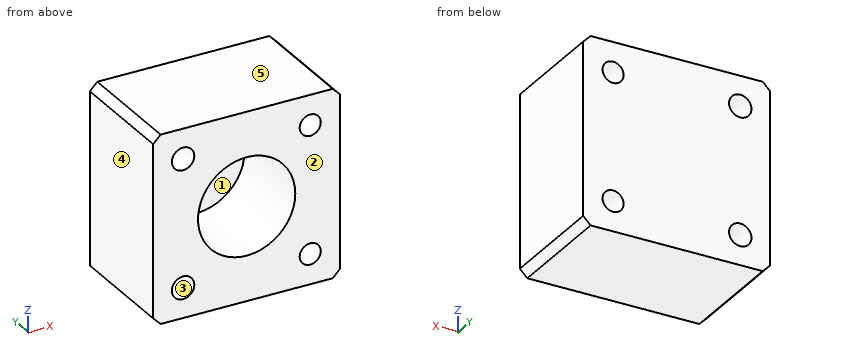
```python
from build123d import *

# Parameters (mm, degrees)
F0_W     = 125
F0_H     = 125
F1_DEPTH = 75
F2_SIZE  = 5
F3_R     = 7.5
F3_R_2   = 7.043913
F4_DEPTH = 75.001
F5_R     = 32.5
F6_DEPTH = 75.001
F7_R     = 32.5
F8_DEPTH = 15


with BuildPart() as f1:
    # F0 (on Front) → F1 (new body)
    with BuildSketch(Plane.XZ):
        Rectangle(F0_W, F0_H)
    extrude(amount=F1_DEPTH)

    # F2
    f2_edges = [f1.edges().sort_by_distance(p)[0] for p in [
        (62.5, -37.5, 62.5),
        (-62.5, -37.5, 62.5),
        (62.5, -37.5, -62.5),
        (-62.5, -37.5, -62.5),
    ]]
    chamfer(f2_edges, length=F2_SIZE)

    # F3 (on face) → F4 (cut, through all)
    with BuildSketch(Plane.XZ.offset(75)):
        with Locations((-42.5, 42.5)):
            Circle(F3_R)
        with Locations((-42.5, -42.5)):
            Circle(F3_R)
        with Locations((42.5, -42.5)):
            Circle(F3_R_2)
        with Locations((42.5, 42.5)):
            Circle(F3_R_2)
    extrude(amount=-F4_DEPTH, mode=Mode.SUBTRACT)

    # F5 (on face) → F6 (cut, through all)
    with BuildSketch(Plane.XZ.offset(75)):
        Circle(F5_R)
    extrude(amount=-F6_DEPTH, mode=Mode.SUBTRACT)

    # F7 (on face) → F8 (join)
    with BuildSketch(Plane(origin=(0, 0, 0), x_dir=(-1, 0, 0), z_dir=(0, 1, 0))):
        Circle(F7_R)
    extrude(amount=-F8_DEPTH)


solid = f1.part
```
Verification items for the finished model (mm, model axes). Face numbers are marked on the shaded views. A direction names the side the tool comes from. Round coordinates to 2 decimals unless told otherwise and drop trailing zeros. Order: outer loops, then holes, each group sorted by start corner. A loop starts at its lowest first (then second) coordinate and runs counter-clockwise, first axis right, second up. Notation, with made-up numbers: (76, -12) - (122, -12) arc R8 ccw to (122, 1) - close; hole circle Ø3 at (-33, -25.75). An arc over 180 degrees is marked (long way). Use CSV: the item, a comma, the result in double quotes.
(1) Section check C-C on y = -27.5. Record the boundary of the cut face in (x, z).
Entries:
outline,"(-62.5, -57.5) - (-57.5, -62.5) - (57.5, -62.5) - (62.5, -57.5) - (62.5, 57.5) - (57.5, 62.5) - (-57.5, 62.5) - (-62.5, 57.5) - close; hole circle Ø15 at (-42.5, -42.5); hole circle Ø15 at (-42.5, 42.5); hole circle Ø65 at (0, 0); hole circle Ø14.09 at (42.5, -42.5); hole circle Ø14.09 at (42.5, 42.5)"
(2) Thickness scan on probe 1 along Z at (x, y) = (-42, -6); probe 2 along Z at (x, y) = (42.5, -55); probe 3 along X at (y, z) = (-28.5, 0). Record the ranges inside material, lowest first. Write a range as from..to.
Entries:
probe 1,"-62.5..-49.98, -35.02..35.02, 49.98..62.5"
probe 2,"-62.5..-49.54, -35.46..35.46, 49.54..62.5"
probe 3,"-62.5..-32.5, 32.5..62.5"
(3) Mould release check, pull along X, two halves, no side actions. Record for the marked faces 3, 4 and 5: released by +X, released by -X, zero draft, split by the parting line, or undercut.
Entries:
face 3,"undercut"
face 4,"released by -X"
face 5,"zero draft"
(4) Access from +Z, -Z, +X, -X, +Y, -Y to the whole of each face (thin tool, end or side, straight path). Record for the marked faces 1 and 2.
Entries:
face 1,"-Y"
face 2,"+Z, -Z, +X, -X, -Y"
(5) Gauge pin test, flat ends, axial feed: pin 1 Ø11.5 at (x, z) = (42.5, -42.5) entering from +Y; pin 2 Ø19.5 at (x, z) = (3.5, 7.5) entering from -Y. Record the tip position at first contact, or that the pin passes through.
Entries:
pin 1,"through"
pin 2,"y = -15"
(6) Section check B-B on z = -42.5. Record the boundary of the cut face in (x, y).
Entries:
outline,"(-62.5, -75) - (-50, -75) - (-50, 0) - (-62.5, 0) - close; (-35, -75) - (35.46, -75) - (35.46, 0) - (-35, 0) - close; (49.54, -75) - (62.5, -75) - (62.5, 0) - (49.54, 0) - close"
(7) Section check A-A on x = -42.5. Record the boundary of the cut face in (y, z).
Entries:
outline,"(-75, -62.5) - (0, -62.5) - (0, -50) - (-75, -50) - close; (-75, -35) - (0, -35) - (0, 35) - (-75, 35) - close; (-75, 50) - (0, 50) - (0, 62.5) - (-75, 62.5) - close"
(8) Section check D-D on y = -10. Record the boundary of the cut face in (x, z).
Entries:
outline,"(-62.5, -57.5) - (-57.5, -62.5) - (57.5, -62.5) - (62.5, -57.5) - (62.5, 57.5) - (57.5, 62.5) - (-57.5, 62.5) - (-62.5, 57.5) - close; hole circle Ø15 at (-42.5, -42.5); hole circle Ø15 at (-42.5, 42.5); hole circle Ø14.09 at (42.5, -42.5); hole circle Ø14.09 at (42.5, 42.5)"
